from build123d import *

# Parameters (mm, degrees)
SKETCH_W        = 63
SKETCH_H        = 45
PAD_DEPTH       = 24
SKETCH001_W     = 61
SKETCH001_H     = 43
POCKET_DEPTH    = 23
SKETCH002_W     = 12
SKETCH002_H     = 7
SKETCH002_W_2   = 9
SKETCH002_H_2   = 10
POCKET001_DEPTH = 2.5
SKETCH003_W     = 16
SKETCH003_H     = 14
POCKET002_DEPTH = 2.5
FILLET_R        = 1
FILLET001_R     = 1
FILLET002_R     = 1
FILLET003_R     = 1
FILLET004_R     = 0.3
FILLET005_R     = 0.3
FILLET006_R     = 0.3
FILLET007_R     = 0.3
FILLET008_R     = 0.3
FILLET009_R     = 0.3


with BuildPart() as part:
    # Sketch → Pad (new body)
    with BuildSketch(Plane.XY):
        Rectangle(SKETCH_W, SKETCH_H)
    extrude(amount=PAD_DEPTH)

    # Sketch001 → Pocket (cut)
    with BuildSketch(Plane.XY.offset(24)):
        Rectangle(SKETCH001_W, SKETCH001_H)
    extrude(amount=-POCKET_DEPTH, mode=Mode.SUBTRACT)

    # Sketch002 → Pocket001 (cut, symmetric)
    with BuildSketch(Plane.YZ.offset(30)):
        with Locations((-5.5, 15.5)):
            Rectangle(SKETCH002_W, SKETCH002_H)
        with Locations((11, 8)):
            Rectangle(SKETCH002_W_2, SKETCH002_H_2)
    extrude(amount=POCKET001_DEPTH, both=True, mode=Mode.SUBTRACT)

    # Sketch003 → Pocket002 (cut, symmetric)
    with BuildSketch(Plane.XZ.offset(-23)):
        with Locations((-0.5, 15)):
            Rectangle(SKETCH003_W, SKETCH003_H)
    extrude(amount=POCKET002_DEPTH, both=True, mode=Mode.SUBTRACT)

    # Fillet
    fillet_edges = [part.edges().sort_by_distance(p)[0] for p in [
        (31.5, 22.5, 12),
    ]]
    fillet(fillet_edges, radius=FILLET_R)

    # Fillet001
    fillet001_edges = [part.edges().sort_by_distance(p)[0] for p in [
        (31.5, -22.5, 12),
    ]]
    fillet(fillet001_edges, radius=FILLET001_R)

    # Fillet002
    fillet002_edges = [part.edges().sort_by_distance(p)[0] for p in [
        (-31.5, -22.5, 12),
    ]]
    fillet(fillet002_edges, radius=FILLET002_R)

    # Fillet003
    fillet003_edges = [part.edges().sort_by_distance(p)[0] for p in [
        (-31.5, 22.5, 12),
    ]]
    fillet(fillet003_edges, radius=FILLET003_R)

    # Fillet004
    fillet004_edges = [part.edges().sort_by_distance(p)[0] for p in [
        (-0.5, 22.5, 8),
    ]]
    fillet(fillet004_edges, radius=FILLET004_R)

    # Fillet005
    fillet005_edges = [part.edges().sort_by_distance(p)[0] for p in [
        (7.5, 22.5, 15),
        (-8.5, 22.5, 15),
    ]]
    fillet(fillet005_edges, radius=FILLET005_R)

    # Fillet006
    fillet006_edges = [part.edges().sort_by_distance(p)[0] for p in [
        (-0.5, 22.5, 22),
    ]]
    fillet(fillet006_edges, radius=FILLET006_R)

    # Fillet007
    fillet007_edges = [part.edges().sort_by_distance(p)[0] for p in [
        (31.5, 11, 3),
        (31.5, 6.5, 8),
        (31.5, 11, 13),
        (31.5, 15.5, 8),
        (31.5, -5.5, 12),
        (31.5, 0.5, 15.5),
        (31.5, -5.5, 19),
        (31.5, -11.5, 15.5),
    ]]
    fillet(fillet007_edges, radius=FILLET007_R)

    # Fillet008
    fillet008_edges = [part.edges().sort_by_distance(p)[0] for p in [
        (-0.5, 21.5, 22),
        (-0.5, 21.5, 8),
        (-8.5, 21.5, 15),
        (7.5, 21.5, 15),
    ]]
    fillet(fillet008_edges, radius=FILLET008_R)

    # Fillet009
    fillet009_edges = [part.edges().sort_by_distance(p)[0] for p in [
        (30.5, 11, 3),
        (30.5, 6.5, 8),
        (30.5, 11, 13),
        (30.5, 15.5, 8),
        (30.5, -5.5, 12),
        (30.5, -11.5, 15.5),
        (30.5, -5.5, 19),
        (30.5, 0.5, 15.5),
    ]]
    fillet(fillet009_edges, radius=FILLET009_R)


solid = part.part
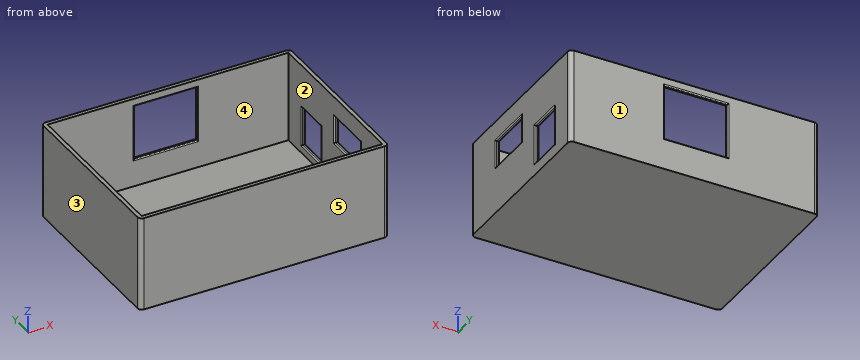
Design review of the part built by this model. Coordinates are the model's own, in mm. Face numbers are marked on the shaded views. A direction names the side the tool comes from. Round coordinates to 2 decimals unless told otherwise and drop trailing zeros. Write each loop counter-clockwise with the first axis right and the second up, starting at its lowest first coordinate (ties: lowest second). Pieces come first, ordered by that corner, then holes. Notation, with made-up numbers: M 49.5,-34.75 L 77.5,-34.75 A16 cw 77.5,-4.75 Z; hole C 83,24.25 d5. An arc over 180 degrees is marked long. One line per item, written item: value. Start each with the question number.
1. Draft analysis for pull direction X (two halves, no side actions). For the marked faces 3, 4 and 5, state which applies: pulls with the +X half, pulls with the -X half, needs draft (parallel to the pull), parting line crosses it, or undercut.
2. Take a section at B-B on y = 11. State the section outline as (x, z) points, then the cut area to 3 significant figures.
3. Take a section at A-A on z = 2. State the section outline as (x, y) points.
4. Take a section at D-D on z = 9.5. State the section outline as (x, y) points, then the cut area to 3 significant figures.
5. To check wall thickness, follow probe 1 along Y at (x, z) = (-17, 5); probe 2 along X at (y, z) = (2, 7); probe 3 along X at (y, z) = (15, 12.75). State the ranges of each line that lie inside material, in increasing order. Write a range as from..to.
6. Take a section at C-C on x = 5. State the section outline as (y, z) points, then the cut area to 3 significant figures.
7. Clearance check with flat-ended pins moving along their axes: P1, Ø12, axis at x = 24, y = 14.5, coming from the -Z side; P2, Ø4, axis at x = -22.5, y = 4, coming from the +Z side. State where each tip first meets the part, or that it passes through.
8. For the marked faces 1 and 2, list the 3-axis set-ups (+Z, -Z, +X, -X, +Y, -Y) from which the entire face can be reached by the end or side of a thin tool; tool diameter is ignored.
Computed:
1. face 3: pulls with the -X half
1. face 4: undercut
1. face 5: needs draft
2. outline: M -31.5,0 L 31.5,0 L 31.5,2.7 A0.3 ccw 31.2,3 L 30.8,3 A0.3 ccw 30.5,2.7 L 30.5,1 L -30.5,1 L -30.5,24 L -31.5,24 Z; M 30.5,13.3 A0.3 ccw 30.8,13 L 31.2,13 A0.3 ccw 31.5,13.3 L 31.5,24 L 30.5,24 Z
2. area: 98.9 mm²
3. outline: M -31.5,-21.5 A1 ccw -30.5,-22.5 L 30.5,-22.5 A1 ccw 31.5,-21.5 L 31.5,21.5 A1 ccw 30.5,22.5 L -30.5,22.5 A1 ccw -31.5,21.5 Z; hole M -30.5,-21.5 L 30.5,-21.5 L 30.5,21.5 L -30.5,21.5 Z
4. outline: M -31.5,-21.5 A1 ccw -30.5,-22.5 L 30.5,-22.5 A1 ccw 31.5,-21.5 L 31.5,6.2 A0.3 ccw 31.2,6.5 L 30.8,6.5 A0.3 ccw 30.5,6.2 L 30.5,-21.5 L -30.5,-21.5 L -30.5,21.5 L -8.8,21.5 A0.3 ccw -8.5,21.8 L -8.5,22.2 A0.3 ccw -8.8,22.5 L -30.5,22.5 A1 ccw -31.5,21.5 Z; M 7.5,21.8 A0.3 ccw 7.8,21.5 L 30.5,21.5 L 30.5,15.8 A0.3 ccw 30.8,15.5 L 31.2,15.5 A0.3 ccw 31.5,15.8 L 31.5,21.5 A1 ccw 30.5,22.5 L 7.8,22.5 A0.3 ccw 7.5,22.2 Z
4. area: 186 mm²
5. probe 1: y = -22.5..-21.5, 21.5..22.5
5. probe 2: x = -31.5..-30.5, 30.5..31.5
5. probe 3: x = -31.5..-30.5
6. outline: M -22.5,0 L 22.5,0 L 22.5,7.7 A0.3 ccw 22.2,8 L 21.8,8 A0.3 ccw 21.5,7.7 L 21.5,1 L -21.5,1 L -21.5,24 L -22.5,24 Z; M 21.5,22.3 A0.3 ccw 21.8,22 L 22.2,22 A0.3 ccw 22.5,22.3 L 22.5,24 L 21.5,24 Z
6. area: 76.9 mm²
7. P1: stops at z = 0
7. P2: stops at z = 1
8. face 1: +Z, -Z, +X, -X, +Y
8. face 2: +Z
